Check sheet for the modelled part. Datum: model origin and axes. Units: mm. A direction names the side the tool comes from. Round coordinates to 2 decimals unless told otherwise and drop trailing zeros. Order: outer loops, then holes, each group sorted by start corner. A loop starts at its lowest first (then second) coordinate and runs counter-clockwise, first axis right, second up. Notation, with made-up numbers: (88, -35) -> (122, -35) arc R14 ccw to (122, -14) -> close; hole circle Ø10 at (25.5, 67.5). An arc over 180 degrees is marked (long way). Answer in a Markdown table with one row per item. Add a question column.
1. Sectioned sample at B-B, the plane x = 16.6. Record the boundary of the cut face in (y, z), then the cut area to 3 significant figures.
2. Depth check by flat-ended pin: P1, Ø0.6, axis at x = -24, z = 7.5, coming from the +Y side; P2, Ø4, axis at x = 28, z = 3.5, coming from the +Y side; P3, Ø0.8, axis at x = -23.5, z = 6, coming from the -Y side; P4, Ø3, axis at x = -16.5, z = 1.5, coming from the +Y side. Enter the tip coordinate at first touch or a pass-through.
3. Material ranges on L1, parallel to Y at x = 0, z = 7.25; L2, parallel to X at y = 7, z = 8; L3, parallel to X at y = -12, z = 6.75, recorded low to high. Write a range as from..to.
4. Sectioned sample at A-A, the plane z = 7.5. Count the separate pieces of the cut face and the enclosed holes in it, then the cut area to 3 significant figures.
5. Sectioned sample at D-D, the plane x = 7. Record the boundary of the cut face in (y, z), then the cut area to 3 significant figures.
6. Draft check along X on faces 1 (the cylindrical face through (-25.95, -6.9, 5.13)), 2 (the flat face through (-28, -7.5, 4)), 3 (the cylindrical face through (-22.15, 21.99, 4.92)). Enter one of: +X half, -X half, draft (parallel to the pull), parting line (faces both ways), or undercut.
7. Sectioned sample at C-C, the plane y = 16.6. Record the boundary of the cut face in (x, z), then the cut area to 3 significant figures.
8. Access from +Z, -Z, +X, -X, +Y, -Y to the whole of each face (thin tool, end or side, straight path). Record for faces 4 (the flat face through (-24, -7.5, 8)), 5 (the cylindrical face through (26.01, 6.93, 6.1)), 6 (the flat face through (19.1, -1.66, 1.23)).
```python
from build123d import *

# Parameters (mm, degrees)
SKETCH1_W           = 50
SKETCH1_H           = 50
SKETCH1_R           = 8
SKETCH1_R_2         = 1.5
BOSS_EXTRUDE1_DEPTH = 9.7
FILLET2_R           = 10
CUT_EXTRUDE1_DEPTH  = 2.5
SKETCH7_W           = 9.7
SKETCH7_H           = 15
BOSS_EXTRUDE2_DEPTH = 5
SKETCH10_W          = 4
SKETCH10_H          = 15
CUT_EXTRUDE2_DEPTH  = 3
FILLET3_R           = 2
CIRPATTERN9_COUNT   = 2
SKETCH11_W          = 4
SKETCH11_H          = 15.220357073
CUT_EXTRUDE3_DEPTH  = 4
FILLET5_R           = 2


with BuildPart() as part:
    # Sketch1 → Boss-Extrude1 (new body)
    with BuildSketch(Plane.XY):
        Rectangle(SKETCH1_W, SKETCH1_H)
        Circle(SKETCH1_R, mode=Mode.SUBTRACT)
        with Locations((16.6, 0)):
            Circle(SKETCH1_R_2, mode=Mode.SUBTRACT)
        with Locations((0, -16.6)):
            Circle(SKETCH1_R_2, mode=Mode.SUBTRACT)
        with Locations((-16.6, 0)):
            Circle(SKETCH1_R_2, mode=Mode.SUBTRACT)
        with Locations((0, 16.6)):
            Circle(SKETCH1_R_2, mode=Mode.SUBTRACT)
    extrude(amount=BOSS_EXTRUDE1_DEPTH)

    # Fillet2
    fillet2_edges = [part.edges().sort_by_distance(p)[0] for p in [
        (-25, -25, 4.85),
        (-25, 25, 4.85),
        (25, 25, 4.85),
        (25, -25, 4.85),
    ]]
    fillet(fillet2_edges, radius=FILLET2_R)

    # Sketch9 → Cut-Extrude1 (cut)
    with BuildSketch(Plane(origin=(0, 0, 0), x_dir=(-1, 0, 0), z_dir=(0, 0, -1))):
        Polygon((2.996447897, -15.020262794), (2.996447897, -18.370262794), (0.095262794, -20.045262794), (-2.805922308, -18.370262794), (-2.805922308, -15.020262794), (0.095262794, -13.345262794), align=None)
        Polygon((18.275, -2.901185103), (14.925, -2.901185103), (13.25, 0), (14.925, 2.901185103), (18.275, 2.901185103), (19.95, 0), align=None)
        Polygon((2.805922308, 14.829737206), (-0.095262794, 13.154737206), (-2.996447897, 14.829737206), (-2.996447897, 18.179737206), (-0.095262794, 19.854737206), (2.805922308, 18.179737206), align=None)
        Polygon((-13.25, -0.190525589), (-14.925, -3.091710692), (-18.275, -3.091710692), (-19.95, -0.190525589), (-18.275, 2.710659514), (-14.925, 2.710659514), align=None)
    extrude(amount=-CUT_EXTRUDE1_DEPTH, mode=Mode.SUBTRACT)

    # Sketch7 → Boss-Extrude2 (add)
    with BuildSketch(Plane(origin=(25, 0, 0), x_dir=(0, 0, -1), z_dir=(1, 0, 0))):
        with Locations((-4.85, 0)):
            Rectangle(SKETCH7_W, SKETCH7_H)
    boss_extrude2 = extrude(amount=BOSS_EXTRUDE2_DEPTH)

    # Sketch10 → Cut-Extrude2 (cut)
    with BuildSketch(Plane.XY.offset(9.7)):
        with Locations((25, 0)):
            Rectangle(SKETCH10_W, SKETCH10_H)
        Polygon((-26.926788745, 7.758740095), (-27.070725077, -7.2405693), (-23.070909239, -7.278952322), (-22.926972907, 7.720357073), align=None)
    extrude(amount=-CUT_EXTRUDE2_DEPTH, mode=Mode.SUBTRACT)

    # Fillet3
    fillet3_edges = [part.edges().sort_by_distance(p)[0] for p in [
        (26, -7.5, 6.7),
        (26, 7.5, 6.7),
    ]]
    fillet(fillet3_edges, radius=FILLET3_R)

    # CirPattern9: Boss-Extrude2 ×2 about axis
    cirpattern9_axis = Axis((0, 0, 0), (0, 0, 1))
    for i in range(1, CIRPATTERN9_COUNT):
        add(boss_extrude2.rotate(cirpattern9_axis, i * 360 / CIRPATTERN9_COUNT))

    # Sketch11 → Cut-Extrude3 (cut)
    with BuildSketch(Plane.XY.offset(9.7)):
        with Locations((-24.926972907, 0.110178536)):
            Rectangle(SKETCH11_W, SKETCH11_H)
    extrude(amount=-CUT_EXTRUDE3_DEPTH, mode=Mode.SUBTRACT)

    # Fillet5
    fillet5_edges = [part.edges().sort_by_distance(p)[0] for p in [
        (-25.963486453, -7.5, 5.7),
        (-25.963486453, 7.5, 5.7),
    ]]
    fillet(fillet5_edges, radius=FILLET5_R)


solid = part.part
```
Answer key:
| question | item | result |
|---|---|---|
| 1 | outline | (-24.87, 0) -> (-3.09, 0) -> (-3.09, 2.5) -> (-1.5, 2.5) -> (-1.5, 9.7) -> (-24.87, 9.7) -> close; (1.5, 2.5) -> (2.71, 2.5) -> (2.71, 0) -> (24.87, 0) -> (24.87, 9.7) -> (1.5, 9.7) -> close |
| 1 | area | 446 mm² |
| 2 | P1 | stops at y = 19.93 |
| 2 | P2 | stops at y = 7.5 |
| 2 | P3 | stops at y = -20.86 |
| 2 | P4 | stops at y = 25 |
| 3 | L1 | y = -25..-18.1, -15.1..-8, 8..15.1, 18.1..25 |
| 3 | L2 | x = -30..-26.93, -22.93..-3.87, 3.87..23, 27..30 |
| 3 | L3 | x = -25..25 |
| 4 | separate pieces | 3 |
| 4 | enclosed holes | 5 |
| 4 | area | 2,210 mm² |
| 5 | outline | (-25, 0) -> (-3.87, 0) -> (-3.87, 9.7) -> (-25, 9.7) -> close; (3.87, 0) -> (25, 0) -> (25, 9.7) -> (3.87, 9.7) -> close |
| 5 | area | 410 mm² |
| 6 | face 1 | undercut |
| 6 | face 2 | draft |
| 6 | face 3 | -X half |
| 7 | outline | (-24.87, 0) -> (-2.81, 0) -> (-2.81, 2.5) -> (-1.5, 2.5) -> (-1.5, 9.7) -> (-24.87, 9.7) -> close; (1.5, 2.5) -> (3, 2.5) -> (3, 0) -> (24.87, 0) -> (24.87, 9.7) -> (1.5, 9.7) -> close |
| 7 | area | 446 mm² |
| 8 | face 4 | +Z |
| 8 | face 5 | +Z, +Y |
| 8 | face 6 | -Z |
